Input: part model. Units: mm. Frame: model coordinates. A direction names the side the tool comes from. Give positions to 0.01 mm unless a question says otherwise; leave off trailing zeros. Loops run counter-clockwise (first coordinate to the right, second up) from the corner with the lowest first, then second, coordinate; pieces in that order, holes last. Notation, with made-up numbers: M -29,86 L 10,86 A7 ccw 10,92 Z; hole C 70,-11 d1. An arc over 180 degrees is marked long. Use CSV: the item, a comma, the result in double quotes. Start each with the question number.
Q1. Section B-B, the plane x = -6. Output: boundary loops of the cut face in (y, z).
Q2. Section A-A, the plane y = -11. Output: boundary loops of the cut face in (x, z).
Q3. Reachability of faces 3 (the cylindrical face through (21.66, 48.94, 1.72)), 4 (the flat face through (41.5, 54, 0)), 5 (the cylindrical face through (-34.85, 48.76, -1.72)), 6 (the flat face through (1, -49.75, 0)) from +Z, -Z, +X, -X, +Y, -Y: full face, straight path, thin tool, end or side. Return the list, or none.
Q4. Pull-direction query (X, two-part tool) for faces 1 (the flat face through (46, 56.75, 0)), 2 (the conical face through (-45.958, -40.741, 0.654)); classes: released by +X, released by -X, zero draft, split by the parting line, or undercut.
Q5. Material intervals for line 1 along X through (y, z) = (41.25, 2.8); line 2 along Y through (x, z) = (21.5, 1.1); line 3 along Y through (x, z) = (-46, 3), sorted ascending.
Q6. Pin query (flat end, axial travel): pin 1 (1.4 mm diameter, centred on x = 29, z = 0, fed in from -Y) (3 decimals); pin 2 (2 mm diameter, centred on x = 35.5, y = 47.75, fed in from -Z); pin 3 (4 mm diameter, centred on x = 29, z = 0, fed in from +Y); pin 4 (4 mm diameter, centred on x = 17.5, z = 0.5, fed in from -Y). Return the tip coordinate at first contact, or that it passes through.
from build123d import *

# Parameters (mm, degrees)
SKETCH1_W           = 100
SKETCH1_H           = 113.5
BOSS_EXTRUDE1_DEPTH = 4.25
CUT_EXTRUDE1_DEPTH  = 77.110528181
M2_HOLE1_C_D        = 2.4
M2_HOLE1_C_DEPTH    = 3
M2_HOLE1_C_TIP      = 0.721032743
M2_HOLE2_D_D        = 2.4
M2_HOLE2_D_DEPTH    = 5
M2_HOLE2_D_TIP      = 0.721032743
M2_HOLE3_E_D        = 2.4
M2_HOLE3_E_DEPTH    = 4
M2_HOLE3_E_TIP      = 0.721032743
M2_HOLE4_F_D        = 2.4
M2_HOLE4_F_DEPTH    = 10
M2_HOLE4_F_TIP      = 0.721032743
M2_HOLE5_G_D        = 2.4
M2_HOLE5_G_DEPTH    = 10
M2_HOLE5_G_TIP      = 0.721032743
M2_HOLE6_H_D        = 2.4
M2_HOLE6_H_DEPTH    = 5
M2_HOLE6_H_TIP      = 0.721032743
FILLET1_R           = 1
CHAMFER1_SIZE       = 1


with BuildPart() as part:
    # Sketch1 → Boss-Extrude1 (new, symmetric)
    with BuildSketch(Plane.XY):
        Rectangle(SKETCH1_W, SKETCH1_H)
    extrude(amount=BOSS_EXTRUDE1_DEPTH, both=True)

    # Sketch4 → Cut-Extrude1 (cut, through all)
    with BuildSketch(Plane.XY.offset(4.25)):
        with BuildLine():
            Line((-40.5, -44.75), (40.5, -44.75))
            ThreePointArc((40.5, -44.75), (41.207106781, -44.457106781), (41.5, -43.75))
            Line((41.5, -43.75), (41.5, 44.25))
            ThreePointArc((41.5, 44.25), (41.207106781, 44.957106781), (40.5, 45.25))
            Line((40.5, 45.25), (-40.5, 45.25))
            ThreePointArc((-40.5, 45.25), (-41.207106781, 44.957106781), (-41.5, 44.25))
            Line((-41.5, 44.25), (-41.5, -43.75))
            ThreePointArc((-41.5, -43.75), (-41.207106781, -44.457106781), (-40.5, -44.75))
        make_face()
        with BuildLine():
            Line((-41.5, 56.75), (41.5, 56.75))
            Line((41.5, 56.75), (41.5, 51.25))
            ThreePointArc((41.5, 51.25), (41.207106781, 50.542893219), (40.5, 50.25))
            Line((40.5, 50.25), (-40.5, 50.25))
            ThreePointArc((-40.5, 50.25), (-41.207106781, 50.542893219), (-41.5, 51.25))
            Line((-41.5, 51.25), (-41.5, 56.75))
        make_face()
        with BuildLine():
            Line((-41.5, -56.75), (41.5, -56.75))
            Line((41.5, -56.75), (41.5, -50.75))
            ThreePointArc((41.5, -50.75), (41.207106781, -50.042893219), (40.5, -49.75))
            Line((40.5, -49.75), (-40.5, -49.75))
            ThreePointArc((-40.5, -49.75), (-41.207106781, -50.042893219), (-41.5, -50.75))
            Line((-41.5, -50.75), (-41.5, -56.75))
        make_face()
    extrude(amount=-CUT_EXTRUDE1_DEPTH, mode=Mode.SUBTRACT)

    # M2 Hole1-C
    with Locations(Plane.XY.offset(4.25)):
        with Locations((-45.75, -40.75), (45.75, -40.75), (-45.75, 41.25), (45.75, 41.25)):
            Hole(M2_HOLE1_C_D / 2, depth=M2_HOLE1_C_DEPTH)
            with Locations((0, 0, -(M2_HOLE1_C_DEPTH + M2_HOLE1_C_TIP / 2))):  # 118° drill point
                Cone(0, M2_HOLE1_C_D / 2, M2_HOLE1_C_TIP, mode=Mode.SUBTRACT)

    # M2 Hole2-D
    with Locations(Plane.XY.offset(4.25)):
        with Locations((-21.5, 47.75), (21.5, 47.75), (-21.5, -47.25), (21.5, -47.25)):
            Hole(M2_HOLE2_D_D / 2, depth=M2_HOLE2_D_DEPTH)
            with Locations((0, 0, -(M2_HOLE2_D_DEPTH + M2_HOLE2_D_TIP / 2))):  # 118° drill point
                Cone(0, M2_HOLE2_D_D / 2, M2_HOLE2_D_TIP, mode=Mode.SUBTRACT)

    # M2 Hole3-E
    with Locations(Plane.XY.offset(4.25)):
        with Locations((0, 47.75), (0, -47.25)):
            Hole(M2_HOLE3_E_D / 2, depth=M2_HOLE3_E_DEPTH)
            with Locations((0, 0, -(M2_HOLE3_E_DEPTH + M2_HOLE3_E_TIP / 2))):  # 118° drill point
                Cone(0, M2_HOLE3_E_D / 2, M2_HOLE3_E_TIP, mode=Mode.SUBTRACT)

    # M2 Hole4-F
    with Locations(Plane(origin=(0, 50.25, 0), x_dir=(1, 0, 0), z_dir=(0, 1, 0))):
        with Locations((-29, 0), (29, 0)):
            Hole(M2_HOLE4_F_D / 2, depth=M2_HOLE4_F_DEPTH)
            with Locations((0, 0, -(M2_HOLE4_F_DEPTH + M2_HOLE4_F_TIP / 2))):  # 118° drill point
                Cone(0, M2_HOLE4_F_D / 2, M2_HOLE4_F_TIP, mode=Mode.SUBTRACT)

    # M2 Hole5-G
    with Locations(Plane(origin=(0, -49.75, 0), x_dir=(-1, 0, 0), z_dir=(0, -1, 0))):
        with Locations((29, 0), (-29, 0)):
            Hole(M2_HOLE5_G_D / 2, depth=M2_HOLE5_G_DEPTH)
            with Locations((0, 0, -(M2_HOLE5_G_DEPTH + M2_HOLE5_G_TIP / 2))):  # 118° drill point
                Cone(0, M2_HOLE5_G_D / 2, M2_HOLE5_G_TIP, mode=Mode.SUBTRACT)

    # M2 Hole6-H
    with Locations(Plane(origin=(0, 0, -4.25), x_dir=(-1, 0, 0), z_dir=(0, 0, -1))):
        with Locations((-35.5, 47.75), (35.5, 47.75), (-35.5, -47.25), (35.5, -47.25)):
            Hole(M2_HOLE6_H_D / 2, depth=M2_HOLE6_H_DEPTH)
            with Locations((0, 0, -(M2_HOLE6_H_DEPTH + M2_HOLE6_H_TIP / 2))):  # 118° drill point
                Cone(0, M2_HOLE6_H_D / 2, M2_HOLE6_H_TIP, mode=Mode.SUBTRACT)

    # Fillet1
    fillet1_edges = [part.edges().sort_by_distance(p)[0] for p in [
        (-50, 0, -4.25),
        (50, 0, -4.25),
    ]]
    fillet(fillet1_edges, radius=FILLET1_R)

    # Chamfer1
    chamfer1_edges = [part.edges().sort_by_distance(p)[0] for p in [
        (-45.75, -56.75, 4.25),
        (45.25, -56.75, -4.25),
        (45.75, -56.75, 4.25),
        (-45.25, -56.75, -4.25),
        (-49.707106781, -56.75, -3.957106781),
        (45.25, 56.75, -4.25),
        (-49.707106781, 56.75, -3.957106781),
        (49.707106781, 56.75, -3.957106781),
        (49.707106781, -56.75, -3.957106781),
        (41.5, -56.75, 0),
        (-41.5, -56.75, 0),
        (-45.25, 56.75, -4.25),
        (-45.75, 56.75, 4.25),
        (-41.5, 56.75, 0),
        (41.5, 56.75, 0),
        (45.75, 56.75, 4.25),
        (50, -56.75, 0.5),
        (-50, -56.75, 0.5),
        (-50, 56.75, 0.5),
        (50, 56.75, 0.5),
    ]]
    chamfer(chamfer1_edges, length=CHAMFER1_SIZE - 0.0001)  # a hair under: the kernel refuses the full size


solid = part.part
A:
1,outline,"M -49.75,-4.25 L -44.75,-4.25 L -44.75,4.25 L -49.75,4.25 Z; M 45.25,-4.25 L 50.25,-4.25 L 50.25,4.25 L 45.25,4.25 Z"
2,outline,"M -50,-3.25 A1 ccw -49,-4.25 L -41.5,-4.25 L -41.5,4.25 L -50,4.25 Z; M 41.5,-4.25 L 49,-4.25 A1 ccw 50,-3.25 L 50,4.25 L 41.5,4.25 Z"
3,face 3,"+Z"
3,face 4,"+Z, -Z, +Y"
3,face 5,"-Z"
3,face 6,"+Z, -Z, -Y"
4,face 1,"zero draft"
4,face 2,"undercut"
5,line 1,"-50 to -46.95, -44.55 to -41.5, 41.5 to 44.55, 46.95 to 50"
5,line 2,"-49.75 to -48.45, -46.05 to -44.75, 45.25 to 46.55, 48.95 to 50.25"
5,line 3,"-56.75 to -41.92, -39.58 to 40.08, 42.42 to 56.75"
6,pin 1,"through"
6,pin 2,"z = 0.87"
6,pin 3,"y = 50.25"
6,pin 4,"y = -49.75"
